```python
from build123d import *

# Parameters (mm, degrees)
EXTRUDE_1_DEPTH     = 20
SKETCH_3_R          = 1.6
CUT_EXTRUDE_2_DEPTH = 41
SKETCH_4_R          = 1.6
CUT_EXTRUDE_3_DEPTH = 41


with BuildPart() as part:
    # Эскиз1 → Бобышка-Вытянуть1 (new body)
    with BuildSketch(Plane.XY):
        Polygon((0, 0), (40, 0), (40, 2), (2, 2), (2, 40), (0, 40), align=None)
    extrude(amount=EXTRUDE_1_DEPTH)

    # Эскиз3 → Вырез-Вытянуть2 (cut, through all)
    with BuildSketch(Plane.ZY):
        with Locations((10, 30)):
            Circle(SKETCH_3_R)
    extrude(amount=-CUT_EXTRUDE_2_DEPTH, mode=Mode.SUBTRACT)

    # Эскиз4 → Вырез-Вытянуть3 (cut, through all)
    with BuildSketch(Plane.XZ):
        with Locations((25, 16)):
            Circle(SKETCH_4_R)
    extrude(amount=-CUT_EXTRUDE_3_DEPTH, mode=Mode.SUBTRACT)


solid = part.part
```
For this review, take the finished solid that the model builds, in its own axes (mm). A direction names the side the tool comes from. Round coordinates to 2 decimals unless told otherwise and drop trailing zeros. Order: outer loops, then holes, each group sorted by start corner. A loop starts at its lowest first (then second) coordinate and runs counter-clockwise, first axis right, second up. Notation, with made-up numbers: (68.25, 41.25) -> (114.25, 41.25) arc R27 cw to (114.25, 67.25) -> close; hole circle Ø8 at (-3.75, -33). An arc over 180 degrees is marked (long way). Use a Markdown table: item, result.
Item 1: Take a section at A-A (z = 10). State the section outline as (x, y) points.
Resolved:
| item | result |
|---|---|
| outline | (0, 0) -> (40, 0) -> (40, 2) -> (2, 2) -> (2, 28.4) -> (0, 28.4) -> close; (0, 31.6) -> (2, 31.6) -> (2, 40) -> (0, 40) -> close |
Item 2: For pin 1 (2.5 mm diameter, centred on x = 25, z = 16, fed in from -Y); pin 2 (2 mm diameter, centred on x = 24, z = 17, fed in from +Y); pin 3 (8 mm diameter, centred on y = 23, z = 7, fed in from +X), all flat-tipped, find the tip position at first contact; note any pin that passes through.
Resolved:
| item | result |
|---|---|
| pin 1 | passes through |
| pin 2 | stops at y = 2 |
| pin 3 | stops at x = 2 |
Item 3: Take a section at D-D (x = 10). State the section outline as (y, z) points, plus the area to 3 significant figures.
Resolved:
| item | result |
|---|---|
| outline | (0, 0) -> (2, 0) -> (2, 20) -> (0, 20) -> close |
| area | 40.0 mm² |
Item 4: Take a section at C-C (z = 2.75). State the section outline as (x, y) points, plus the area to 3 significant figures.
Resolved:
| item | result |
|---|---|
| outline | (0, 0) -> (40, 0) -> (40, 2) -> (2, 2) -> (2, 40) -> (0, 40) -> close |
| area | 156 mm² |
Item 5: Take a section at B-B (y = 30). State the section outline as (x, z) points, plus the area to 3 significant figures.
Resolved:
| item | result |
|---|---|
| outline | (0, 0) -> (2, 0) -> (2, 8.4) -> (0, 8.4) -> close; (0, 11.6) -> (2, 11.6) -> (2, 20) -> (0, 20) -> close |
| area | 33.6 mm² |
Item 6: For line 1 along Y through (x, z) = (0.7, 10); line 2 along Z through (x, y) = (25, 1); line 3 along X through (y, z) = (20.5, 12.25), list the stretches that pass through material, from the lowest coordinate up. Write a range as [from, to].
Resolved:
| item | result |
|---|---|
| line 1 | y = [0, 28.4], [31.6, 40] |
| line 2 | z = [0, 14.4], [17.6, 20] |
| line 3 | x = [0, 2] |
Item 7: Machinability: for faces 5 (the flat face through (21, 2, 10)), 6 (the flat face through (1, 11, 20)), which of the approach directions +Z, -Z, +X, -X, +Y, -Y give a long, thin tool a straight path to every point of the face, cutting with its end or side? Answer none if there is none.
Resolved:
| item | result |
|---|---|
| face 5 | +Z, -Z, +X, +Y |
| face 6 | +Z, +X, -X, +Y, -Y |
Item 8: Draft analysis for pull direction Z (two halves, no side actions). For faces 1 (the cylindrical face through (24.792, 0.986, 17.586)), 2 (the cylindrical face through (0.99, 31.08, 8.82)), 3 (the flat face through (1, 11, 0)), 4 (the flat face through (40, 1, 10)), state which applies: +Z half, -Z half, draft (parallel to the pull), parting line (faces both ways), or undercut.
Resolved:
| item | result |
|---|---|
| face 1 | undercut |
| face 2 | undercut |
| face 3 | -Z half |
| face 4 | draft |
